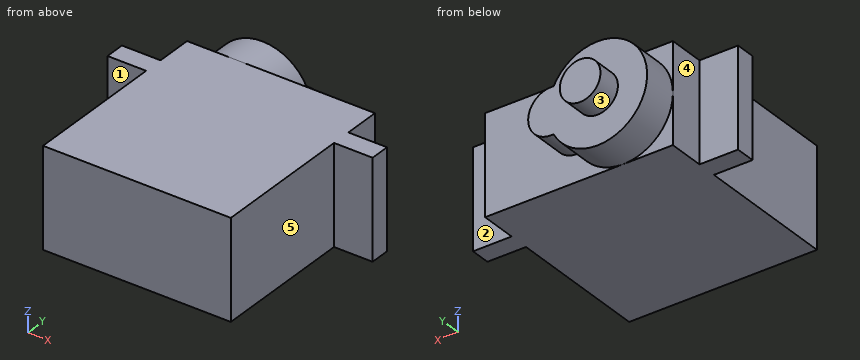
from build123d import *

# Parameters (mm, degrees)
BOSS_EXTRUDE1_DEPTH = 12.065
BOSS_EXTRUDE2_DEPTH = 4.318
SKETCH3_R           = 2.4765
BOSS_EXTRUDE3_DEPTH = 2.921


with BuildPart() as part:
    # Sketch1 → Boss-Extrude1 (new body)
    with BuildSketch(Plane.XY):
        Polygon((0, 0), (22.86, 0), (22.86, 17.272), (27.559, 17.272), (27.559, 19.685), (22.86, 19.685), (22.86, 24.13), (0, 24.13), (0, 19.685), (-4.699, 19.685), (-4.699, 17.272), (0, 17.272), align=None)
    extrude(amount=BOSS_EXTRUDE1_DEPTH)

    # Sketch2 → Boss-Extrude2 (add)
    with BuildSketch(Plane(origin=(0, 24.13, 0), x_dir=(1, 0, 0), z_dir=(0, 1, 0))):
        with BuildLine():
            ThreePointArc((11.387191011, -8.810690135), (14.478, -6.0325), (11.387191011, -3.254309865))
            ThreePointArc((11.387191011, -3.254309865), (0, -6.0325), (11.387191011, -8.810690135))
        make_face()
    extrude(amount=BOSS_EXTRUDE2_DEPTH)

    # Sketch3 → Boss-Extrude3 (add)
    with BuildSketch(Plane(origin=(0, 28.448, 0), x_dir=(1, 0, 0), z_dir=(0, 1, 0))):
        with Locations((6.0325, -6.0325)):
            Circle(SKETCH3_R)
    extrude(amount=BOSS_EXTRUDE3_DEPTH)


solid = part.part
Verification items for the finished model (mm, model axes). Face numbers are marked on the shaded views. A direction names the side the tool comes from. Coordinates: 2 decimals unless noted, no trailing zeros. Loops run counter-clockwise (first coordinate to the right, second up) from the corner with the lowest first, then second, coordinate; pieces in that order, holes last. Notation, with made-up numbers: (7, 55.25) -> (51, 55.25) arc R7 cw to (51, 66.25) -> close; hole circle Ø10 at (-15.75, -8.75). An arc over 180 degrees is marked (long way). Answer as a JSON object with one key per item and string values. Group by question number.
Item 1: Sectioned sample at C-C on y = 16.5. Record the boundary of the cut face in (x, z) (3 decimals).
Item 2: Tool access check on the marked faces 1, 2, 3, 4 and 5. Record the directions out of +Z, -Z, +X, -X, +Y, -Y that give a thin tool (end or side, any length) a straight path to the whole face; none if there is none.
Item 3: Scan lines: probe 1 along Y at (x, z) = (9.5, 2); probe 2 along Y at (x, z) = (21, 10.5); probe 3 along X at (y, z) = (21.5, 5.75). Record each from-to range of solid material in increasing order.
Item 4: Sectioned sample at B-B on x = 13. Record the boundary of the cut face in (y, z) (3 decimals).
Item 5: Sectioned sample at A-A on z = 7.25. Record the boundary of the cut face in (x, y) (3 decimals).
Item 6: Depth check by flat-ended pin: pin 1 (3.5 mm diameter, centred on y = 21.5, z = 5, fed in from -X); pin 2 (5 mm diameter, centred on x = -3, z = 5.5, fed in from -Y); pin 3 (3 mm diameter, centred on x = 3.5, z = 2.5, fed in from +Y); pin 4 (3 mm diameter, centred on x = 16, z = 4.5, fed in from -Y). Enter the tip coordinate at first touch or a pass-through.
Item 7: Sectioned sample at D-D on z = 11. Record the boundary of the cut face in (x, y) (3 decimals).
Evaluation:
{
 "1": {"outline": "(0, 0) -> (22.86, 0) -> (22.86, 12.065) -> (0, 12.065) -> close"},
 "2": {"face 1": "+Z, -Z, -X, -Y", "face 2": "+Z, -Z, +X, +Y", "face 3": "+Y", "face 4": "+Z, -Z, -X, +Y", "face 5": "+Z, -Z, +X, -Y"},
 "3": {"probe 1": "y = 0 to 28.45", "probe 2": "y = 0 to 24.13", "probe 3": "x = 0 to 22.86"},
 "4": {"outline": "(0, 0) -> (24.13, 0) -> (24.13, 3.568) -> (28.448, 3.568) -> (28.448, 8.497) -> (24.13, 8.497) -> (24.13, 12.065) -> (0, 12.065) -> close"},
 "5": {"outline": "(-4.699, 17.272) -> (0, 17.272) -> (0, 0) -> (22.86, 0) -> (22.86, 17.272) -> (27.559, 17.272) -> (27.559, 19.685) -> (22.86, 19.685) -> (22.86, 24.13) -> (14.199, 24.13) -> (14.199, 28.448) -> (8.189, 28.448) -> (8.189, 31.369) -> (3.876, 31.369) -> (3.876, 28.448) -> (0.124, 28.448) -> (0.124, 24.13) -> (0, 24.13) -> (0, 19.685) -> (-4.699, 19.685) -> close"},
 "6": {"pin 1": "stops at x = 0", "pin 2": "stops at y = 17.27", "pin 3": "stops at y = 28.45", "pin 4": "stops at y = 0"},
 "7": {"outline": "(-4.699, 17.272) -> (0, 17.272) -> (0, 0) -> (22.86, 0) -> (22.86, 17.272) -> (27.559, 17.272) -> (27.559, 19.685) -> (22.86, 19.685) -> (22.86, 24.13) -> (9.455, 24.13) -> (9.455, 28.448) -> (2.61, 28.448) -> (2.61, 24.13) -> (0, 24.13) -> (0, 19.685) -> (-4.699, 19.685) -> close"}
}
